from build123d import *

# Parameters (mm, degrees)
F0_W           = 150
F0_H           = 200
F1_DEPTH       = 10
F3_D           = 5
F5_DEPTH       = 10
F6_DEPTH       = 10
F7_D           = 6.6
F7_CBORE_D     = 11.25
F7_CBORE_DEPTH = 6
F8_D           = 5.5
F8_CBORE_D     = 9.75
F8_CBORE_DEPTH = 5


# Not quite as in the source:
# - a feature names something its author has since deleted; it is built from what else it names


with BuildPart() as f1:
    # F0 (on Top) → F1 (new body)
    with BuildSketch(Plane.XY):
        with Locations((34.3934863061, 53.7353821645)):
            Rectangle(F0_W, F0_H)
    extrude(amount=F1_DEPTH)

    # F3 (through all)
    with Locations(Plane(origin=(0, 0, 0), x_dir=(1, 0, 0), z_dir=(0, 0, -1))):
        with Locations((-31.1065136939, -140.7353821645), (-31.1065136939, -114.7353821645), (-31.1065136939, -88.7353821645), (99.8934863061, -88.7353821645), (99.8934863061, -114.7353821645), (99.8934863061, -140.7353821645)):
            Hole(F3_D / 2)

    # F5 (add): a face of the model
    f5_faces = [f1.faces().sort_by_distance(p)[0] for p in [
        (109.3934863061, 53.7353821645, 5),
    ]]
    extrude(f5_faces, amount=F5_DEPTH)

    # F6 (add): a face of the model
    f6_faces = [f1.faces().sort_by_distance(p)[0] for p in [
        (-40.6065136939, 53.7353821645, 5),
    ]]
    extrude(f6_faces, amount=F6_DEPTH)

    # F7 (through all)
    with Locations(Plane(origin=(0, 0, 0), x_dir=(1, 0, 0), z_dir=(0, 0, -1))):
        with Locations((-37.1065136939, 36.2646178355), (-37.1065136939, 6.2646178355), (105.8934863061, 36.2646178355), (105.8934863061, 6.2646178355), (105.8934863061, -35.7353821645), (105.8934863061, -65.7353821645), (-37.1065136939, -65.7353821645), (-37.1065136939, -35.7353821645)):
            CounterBoreHole(F7_D / 2, F7_CBORE_D / 2, F7_CBORE_DEPTH)

    # F8 (through all)
    with Locations(Plane(origin=(0, 0, 0), x_dir=(1, 0, 0), z_dir=(0, 0, -1))):
        with Locations((54.8934863061, -51.2353821645), (54.8934863061, -66.2353821645), (14.8934863061, -51.2353821645), (14.8934863061, -66.2353821645)):
            CounterBoreHole(F8_D / 2, F8_CBORE_D / 2, F8_CBORE_DEPTH)


solid = f1.part
Model file for the job. Use its own axes, mm. A direction names the side the tool comes from. Coordinates: 2 decimals unless noted, no trailing zeros. Write each question's results on one line, items separated by ' | '. Start each with the question number.
1) Cut at A-A (z = 3). Count the separate pieces of the cut face and the enclosed holes in it, then the cut area to 3 significant figures.
2) 3-axis set-ups, long thin cutter, end or side, ignore diameter. For faces 1 (the face through (17, 53.3, 5)), 2 (the face through (-36.391, 68.957, 8.028)): which of +Z, -Z, +X, -X, +Y, -Y reach the whole face in a straight line?
3) Probe line 1 along Y through (x, z) = (100, 9); line 2 along X through (y, z) = (51, 6); line 3 along Y through (x, z) = (-32, 6.5). List the from-to ranges inside material, lowest first. Write a range as from..to.
4) Mould opens along X. For faces 3 (the face through (53.837, 55.994, 2.465)), 4 (the face through (36, 52, 10)), 5 (the face through (17.64, 51.11, 7.54)) say: pulls with the +X half, pulls with the -X half, needs draft (parallel to the pull), parting line crosses it, or undercut.
5) Flat gauge pins, fed straight in: P1, Ø11, axis at x = 54.89, y = 66.24, coming from the +Z side; P2, Ø5.5, axis at x = -35.5, y = 35, coming from the -Z side. Where does each tip first touch, or does it go through?
Returned:
1) separate pieces: 1 | enclosed holes: 18 | area: 32,800 mm^2
2) face 1: -Z | face 2: +Z, -Z
3) line 1: -46.26..86.24, 91.23..112.24, 117.23..138.24, 143.23..153.74 | line 2: -50.61..12.15, 17.63..52.15, 57.63..119.39 | line 3: -46.26..86.4, 91.07..112.4, 117.07..138.4, 143.07..153.74
4) face 3: undercut | face 4: needs draft | face 5: undercut
5) P1: z = 10 | P2: z = 6
